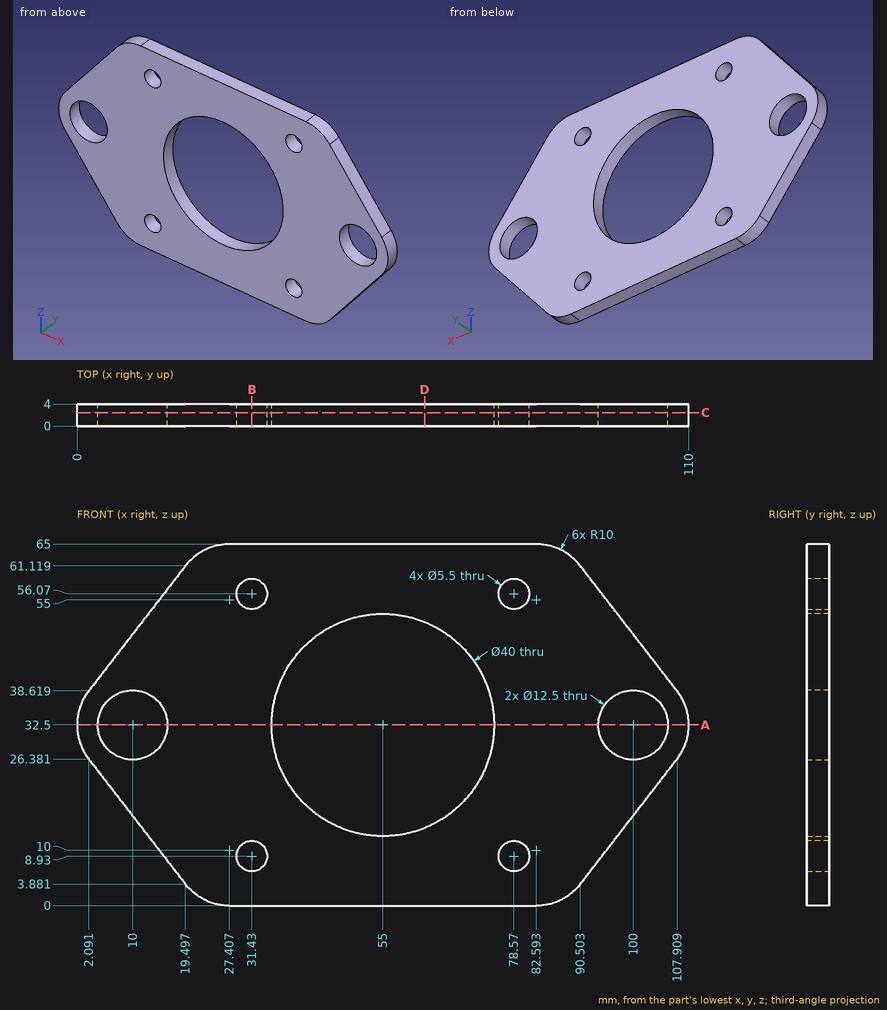
The drawing under review shows one solid part. Ordinate dimensions are in mm from its lowest x, y, z. Round coordinates to 2 decimals unless told otherwise and drop trailing zeros. Order: outer loops, then holes, each group sorted by start corner. A loop starts at its lowest first (then second) coordinate and runs counter-clockwise, first axis right, second up. Notation, with made-up numbers: M -26,-11 L 1,-11 A23 cw 1,0 Z; hole C -22,14.25 d4. An arc over 180 degrees is marked long. Answer as CSV lines item,"result". Start each with the question number.
1) Wall thickness on line 1 along X through (y, z) = (3.2, 32.5); line 2 along Z through (x, y) = (80.5, 1.2); line 3 along X through (y, z) = (1.3, 8.93): over which ranges is each line inside the solid? List them lowest first. Write a range as [from, to].
2) Add section C-C (y = 2.45). Give the boundary of the cut face in (x, z).
3) For pin 1 Ø2 at (y, z) = (1.5, 7) entering from -X; pin 2 Ø2 at (x, y) = (90, 1) entering from +Z, all flat-tipped, find the tip position at first contact; note any pin that passes through.
4) Add section B-B (x = 31.43). Give the boundary of the cut face in (y, z).
5) Add section A-A (z = 32.5). Give the boundary of the cut face in (x, y), then the cut area to 3 significant figures.
6) Add section D-D (x = 62.5). Give the boundary of the cut face in (y, z), then the cut area to 3 significant figures.
Resolved:
1,line 1,"[0, 3.75], [16.25, 35], [75, 93.75], [106.25, 110]"
1,line 2,"[0, 6.97], [10.89, 54.11], [58.03, 65]"
1,line 3,"[15.59, 28.68], [34.18, 75.82], [81.32, 94.41]"
2,outline,"M 2.09,26.38 L 19.5,3.88 A10 ccw 27.41,0 L 82.59,0 A10 ccw 90.5,3.88 L 107.91,26.38 A10 ccw 107.91,38.62 L 90.5,61.12 A10 ccw 82.59,65 L 27.41,65 A10 ccw 19.5,61.12 L 2.09,38.62 A10 ccw Z; hole C 10,32.5 d12.5; hole C 31.43,8.93 d5.5; hole C 31.43,56.07 d5.5; hole C 55,32.5 d40; hole C 78.57,8.93 d5.5; hole C 78.57,56.07 d5.5; hole C 100,32.5 d12.5"
3,pin 1,"x = 16.31"
3,pin 2,"z = 62.68"
4,outline,"M 0,0 L 4,0 L 4,6.18 L 0,6.18 Z; M 0,11.68 L 4,11.68 L 4,53.32 L 0,53.32 Z; M 0,58.82 L 4,58.82 L 4,65 L 0,65 Z"
5,outline,"M 0,0 L 3.75,0 L 3.75,4 L 0,4 Z; M 16.25,0 L 35,0 L 35,4 L 16.25,4 Z; M 75,0 L 93.75,0 L 93.75,4 L 75,4 Z; M 106.25,0 L 110,0 L 110,4 L 106.25,4 Z"
5,area,"180 mm^2"
6,outline,"M 0,0 L 4,0 L 4,13.96 L 0,13.96 Z; M 0,51.04 L 4,51.04 L 4,65 L 0,65 Z"
6,area,"112 mm^2"
